Read the model definition and answer for the solid it produces. Units are mm, in the model's axes. Face numbers are marked on the shaded views. A direction names the side the tool comes from. Coordinates: 2 decimals unless noted, no trailing zeros. Loops run counter-clockwise (first coordinate to the right, second up) from the corner with the lowest first, then second, coordinate; pieces in that order, holes last. Notation, with made-up numbers: M -22,78.25 L 25,78.25 A19 cw 25,106.25 Z; hole C 30.25,79 d3. An arc over 180 degrees is marked long. One line per item, written item: value. Start each with the question number.
1. Consider probe 1 along Y at (x, z) = (31, 8.75); probe 2 along Y at (x, z) = (-39.5, 2); probe 3 along X at (y, z) = (-2, 7.5). Determine where each line is inside the solid, lowest interval first.
2. The part is cut by section B-B (x = -35). Write down the section's boundary in (y, z).
3. The part is cut by section A-A (y = 0). Write down the section's boundary in (x, z), then the cut area to 4 significant figures.
4. For the marked faces 1 and 2, determine the directions among +Z, -Z, +X, -X, +Y, -Y from which every point of the face is accessible in a straight line to the end or side of a thin tool.
5. The part is cut by section C-C (x = 0). State how many separate pieces and enclosed holes the cut face has, then the cut area to 3 significant figures.
6. Flat-ended cylindrical pins translate along their axes: pin 1 (4 mm diameter, centred on x = 21.65, y = 12.5, fed in from -Z); pin 2 (1.5 mm diameter, centred on y = 31, z = 7, fed in from -X); pin 3 (8 mm diameter, centred on x = 21.65, y = -12.5, fed in from +Z); pin 4 (1.5 mm diameter, centred on y = 13, z = 11, fed in from +X). Find the tip coordinate at first contact, or state that the pin passes through.
Autodesk Inventor part; units mm, degrees
ref_plane "YZ Plane" through (0, 0, 0) normal (1, 0, 0) x (0, 1, 0)
ref_plane "XZ Plane" through (0, 0, 0) normal (0, 1, 0) x (-1, 0, 0)
ref_plane "XY Plane" through (0, 0, 0) normal (0, 0, 1) x (1, 0, 0)
sketch "Sketch2" plane through (0, 0, 0) normal (0, 0, 1) x (1, 0, 0)
  circle A0 centre (0, 0) radius 62.5
  circle A1 centre (0, 0) radius 2.5
  dimension "d0" = 125
  dimension "d1" = 5
extrude "Extrusion1" add sketch "Sketch2" along normal blind 15
sketch "Sketch4" plane through (0, 0, 0) normal (0, 0, -1) x (-1, 0, 0)
  circle A0 centre (0, 25) radius 2.575
  circle A1 centre (-21.6506, 12.5) radius 2.575
  circle A2 centre (-21.6506, -12.5) radius 2.575
  circle A3 centre (0, -25) radius 2.575
  circle A4 centre (21.6506, -12.5) radius 2.575
  circle A5 centre (21.6506, 12.5) radius 2.575
  point P0 (0, 0)
  dimension "d8" = 5.15
  dimension "d9" = 25
  dimension "d12" = 360
extrude "Extrusion3" cut sketch "Sketch4" against normal through all
sketch "Sketch5" plane through (0, 0, 15) normal (0, 0, 1) x (1, 0, 0)
  circle A0 centre (0, 0) radius 37.5
  dimension "d16" = 75
extrude "Extrusion4" cut sketch "Sketch5" against normal blind 5
sketch "Sketch6" plane through (0, 0, 15) normal (0, 0, 1) x (1, 0, 0)
  circle A0 centre (0, 55) radius 2.5
  circle A1 centre (-47.6314, 27.5) radius 2.5
  circle A2 centre (-47.6314, -27.5) radius 2.5
  circle A3 centre (0, -55) radius 2.5
  circle A4 centre (47.6314, -27.5) radius 2.5
  circle A5 centre (47.6314, 27.5) radius 2.5
  point P0 (0, 0)
  dimension "d19" = 5
  dimension "d20" = 55
  dimension "d23" = 360
extrude "Extrusion5" cut sketch "Sketch6" against normal through all
sketch "Sketch8" plane through (0, 0, 15) normal (0, 0, 1) x (1, 0, 0)
  circle A0 centre (0, 0) radius 37.5
  circle A1 centre (0, 0) radius 62.5
  circle A2 centre (0, 55) radius 2.5
  circle A3 centre (0, 55) radius 5
  circle A4 centre (-47.6314, 27.5) radius 5
  circle A5 centre (-47.6314, -27.5) radius 5
  circle A6 centre (0, -55) radius 5
  circle A7 centre (47.6314, -27.5) radius 5
  circle A8 centre (47.6314, 27.5) radius 5
  point P0 (-56.2917, 32.5)
  point P1 (-56.2917, -32.5)
  point P2 (0, -65)
  point P3 (56.2917, -32.5)
  point P4 (56.2917, 32.5)
  dimension "d28" = 10
  dimension "d31" = 360
extrude "Extrusion6" cut sketch "Sketch8" against normal blind 5 contours A2 | A3 | A4 | A5 | A6 | A7 | A8
sketch "Sketch9" plane through (0, 0, 15) normal (0, 0, 1) x (1, 0, 0)
  circle A0 centre (0, 0) radius 2.5 construction
  circle A1 centre (0, 0) radius 42.5 construction
  circle A2 centre (0, 0) radius 57.5 construction
  line L0 (40.4629, 13) -> (54.61, 18)
  line L1 (40.4629, -13) -> (54.61, -18)
  line L2 (0, 0) -> (92.9665, 0) construction
  arc A3 (40.4629, -13) -> (40.4629, 13) centre (0, 0) ccw
  arc A4 (54.61, -18) -> (54.61, 18) centre (0, 0) ccw
  circle A5 centre (0, 0) radius 42.5 construction
  line L3 (8.9731, 41.5419) -> (11.7165, 56.2936)
  arc A6 (31.4898, 28.5419) -> (8.9731, 41.5419) centre (0, 0) ccw
  line L4 (31.4898, 28.5419) -> (42.8934, 38.2936)
  circle A7 centre (0, 0) radius 57.5 construction
  arc A8 (42.8934, 38.2936) -> (11.7165, 56.2936) centre (0, 0) ccw
  circle A9 centre (0, 0) radius 42.5 construction
  line L5 (-31.4898, 28.5419) -> (-42.8934, 38.2936)
  arc A10 (-8.9731, 41.5419) -> (-31.4898, 28.5419) centre (0, 0) ccw
  line L6 (-8.9731, 41.5419) -> (-11.7165, 56.2936)
  circle A11 centre (0, 0) radius 57.5 construction
  arc A12 (-11.7165, 56.2936) -> (-42.8934, 38.2936) centre (0, 0) ccw
  circle A13 centre (0, 0) radius 42.5 construction
  line L7 (-40.4629, -13) -> (-54.61, -18)
  arc A14 (-40.4629, 13) -> (-40.4629, -13) centre (0, 0) ccw
  line L8 (-40.4629, 13) -> (-54.61, 18)
  circle A15 centre (0, 0) radius 57.5 construction
  arc A16 (-54.61, 18) -> (-54.61, -18) centre (0, 0) ccw
  circle A17 centre (0, 0) radius 42.5 construction
  line L9 (-8.9731, -41.5419) -> (-11.7165, -56.2936)
  arc A18 (-31.4898, -28.5419) -> (-8.9731, -41.5419) centre (0, 0) ccw
  line L10 (-31.4898, -28.5419) -> (-42.8934, -38.2936)
  circle A19 centre (0, 0) radius 57.5 construction
  arc A20 (-42.8934, -38.2936) -> (-11.7165, -56.2936) centre (0, 0) ccw
  circle A21 centre (0, 0) radius 42.5 construction
  line L11 (31.4898, -28.5419) -> (42.8934, -38.2936)
  arc A22 (8.9731, -41.5419) -> (31.4898, -28.5419) centre (0, 0) ccw
  line L12 (8.9731, -41.5419) -> (11.7165, -56.2936)
  circle A23 centre (0, 0) radius 57.5 construction
  arc A24 (11.7165, -56.2936) -> (42.8934, -38.2936) centre (0, 0) ccw
  dimension "d35" = 85
  dimension "d36" = 115
  dimension "d37" = 13
  dimension "d38" = 18
  dimension "d41" = 360
extrude "Extrusion7" cut sketch "Sketch9" against normal through all
properties part number "SJ002" material "ABS Plastic"
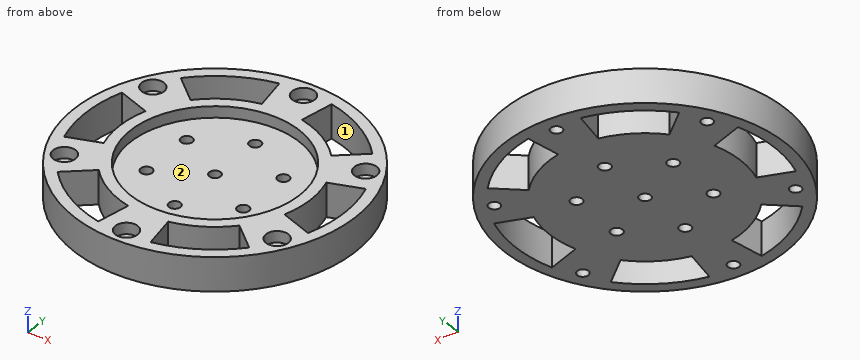
Answer block:
1. probe 1: y = -54.27 to -48.43, -29.07 to 29.07, 48.43 to 54.27
1. probe 2: y = -48.44 to -41.79, -35.39 to 35.39, 41.79 to 48.44
1. probe 3: x = -62.47 to -57.47, -42.45 to -1.5, 1.5 to 42.45, 57.47 to 62.47
2. outline: M -51.78,0 L -45.62,0 L -45.62,15 L -51.78,15 Z; M -31.54,0 L 31.54,0 L 31.54,15 L 13.46,15 L 13.46,10 L -13.46,10 L -13.46,15 L -31.54,15 Z; M 45.62,0 L 51.78,0 L 51.78,15 L 45.62,15 Z
3. outline: M -62.5,0 L -57.5,0 L -57.5,15 L -62.5,15 Z; M -42.5,0 L -2.5,0 L -2.5,10 L -37.5,10 L -37.5,15 L -42.5,15 Z; M 2.5,0 L 42.5,0 L 42.5,15 L 37.5,15 L 37.5,10 L 2.5,10 Z; M 57.5,0 L 62.5,0 L 62.5,15 L 57.5,15 Z
3. area: 1,000 mm2
4. face 1: +Z, -Z
4. face 2: +Z
5. separate pieces: 6
5. enclosed holes: 0
5. area: 1,150 mm2
6. pin 1: passes through
6. pin 2: stops at x = -54.69
6. pin 3: stops at z = 10
6. pin 4: stops at x = 61.29
